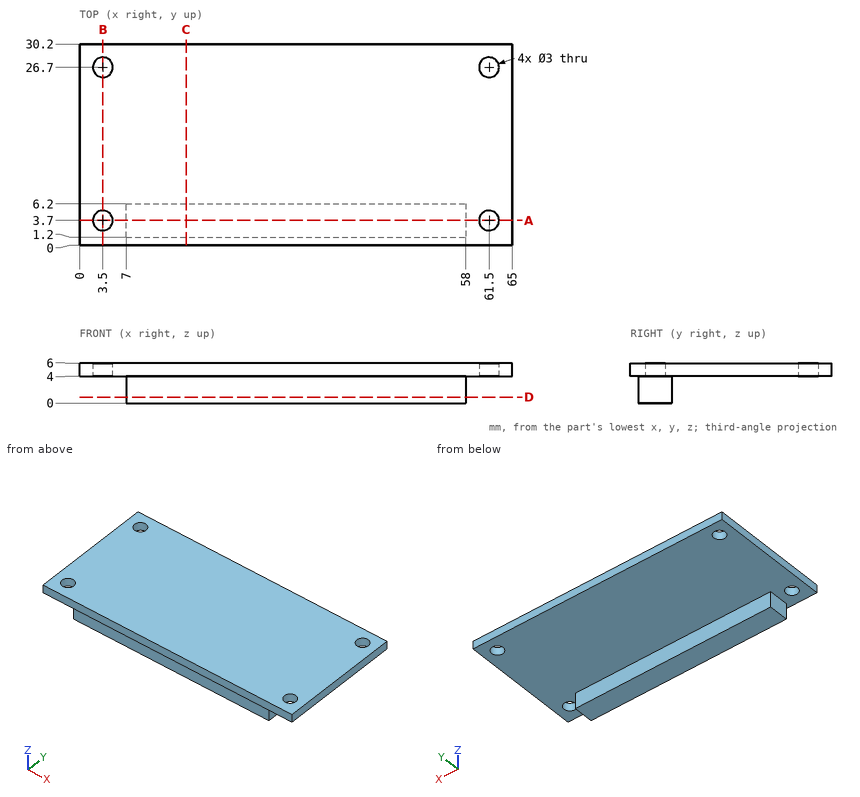
Input: dimensioned drawing with shaded views. Units: mm. Origin: part minimum x, y, z. Round coordinates to 2 decimals unless told otherwise and drop trailing zeros. Order: outer loops, then holes, each group sorted by start corner. A loop starts at its lowest first (then second) coordinate and runs counter-clockwise, first axis right, second up. Notation, with made-up numbers: (87.25, -19.5) - (100.25, -19.5) arc R29 cw to (100.25, 11.5) - close; hole circle Ø10 at (56.25, 6). An arc over 180 degrees is marked (long way). Answer as a JSON object with one key per item and string values. Group by question number.
(1) Cut plane A-A (y = 3.7). Return loops of the section in (x, z), then the cut area to 3 significant figures.
(2) Cut plane D-D (z = 0.9). Return loops of the section in (x, y), then the cut area to 3 significant figures.
(3) Cut plane C-C (x = 16). Return loops of the section in (y, z).
(4) Cut plane B-B (x = 3.5). Return loops of the section in (y, z), then the cut area to 3 significant figures.
(5) Pin query (flat end, axial travel): P1, Ø2.5, axis at x = 3.5, y = 26.7, coming from the -Z side; P2, Ø1, axis at x = 14, y = 17.5, coming from the -Z side; P3, Ø1.2, axis at y = 4.5, z = 2.5, coming from the +X side. Return the tip coordinate at first contact, or that it passes through.
(6) Material intervals for probe 1 along Y at (x, z) = (61.5, 4.85); probe 2 along Y at (x, z) = (62.5, 5.05); probe 3 along X at (y, z) = (2.5, 4.15), sorted ascending. Write a range as from..to.
Here are the results:
{
 "1": {"outline": "(0, 4) - (2, 4) - (2, 6) - (0, 6) - close; (5, 4) - (7, 4) - (7, 0) - (58, 0) - (58, 4) - (60, 4) - (60, 6) - (5, 6) - close; (63, 4) - (65, 4) - (65, 6) - (63, 6) - close", "area": "322 mm^2"},
 "2": {"outline": "(7, 1.2) - (58, 1.2) - (58, 6.2) - (7, 6.2) - close", "area": "255 mm^2"},
 "3": {"outline": "(0, 4) - (1.2, 4) - (1.2, 0) - (6.2, 0) - (6.2, 4) - (30.2, 4) - (30.2, 6) - (0, 6) - close"},
 "4": {"outline": "(0, 4) - (2.2, 4) - (2.2, 6) - (0, 6) - close; (5.2, 4) - (25.2, 4) - (25.2, 6) - (5.2, 6) - close; (28.2, 4) - (30.2, 4) - (30.2, 6) - (28.2, 6) - close", "area": "48.4 mm^2"},
 "5": {"P1": "passes through", "P2": "stops at z = 4", "P3": "stops at x = 58"},
 "6": {"probe 1": "y = 0..2.2, 5.2..25.2, 28.2..30.2", "probe 2": "y = 0..2.58, 4.82..25.58, 27.82..30.2", "probe 3": "x = 0..2.6, 4.4..60.6, 62.4..65"}
}
